from build123d import *

# Parameters (mm, degrees)
F0_W     = 20
F0_H     = 15
F0_W_2   = 75
F0_H_2   = 35
F0_W_3   = 15
F1_DEPTH = 60
F3_DEPTH = 50


with BuildPart() as f1:
    # F0 (on Top) → F1 (new body)
    with BuildSketch(Plane.XY):
        with Locations((45, 17.5)):
            Rectangle(F0_W, F0_H)
        with Locations((-2.5, 17.5)):
            Rectangle(F0_W_2, F0_H)
        with Locations((45, -7.5)):
            Rectangle(F0_W, F0_H_2)
        with Locations((-47.5, 17.5)):
            Rectangle(F0_W_3, F0_H)
        with Locations((-47.5, -7.5)):
            Rectangle(F0_W_3, F0_H_2)
    extrude(amount=F1_DEPTH)

    # F2 (on face) → F3 (cut)
    with BuildSketch(Plane.XZ.offset(25)):
        Polygon((55, 60), (-15, 60), (55, 20), align=None)
    extrude(amount=-F3_DEPTH, mode=Mode.SUBTRACT)


solid = f1.part
Source: CAD feature listing. Evaluate the final solid. Frame: model axes, mm. A direction names the side the tool comes from. Round coordinates to 2 decimals unless told otherwise and drop trailing zeros. Write each loop counter-clockwise with the first axis right and the second up, starting at its lowest first coordinate (ties: lowest second). Pieces come first, ordered by that corner, then holes. Notation, with made-up numbers: (9.5, -27.5) - (16.5, -27.5) arc R15 ccw to (16.5, -5.5) - close; hole circle Ø11 at (-6.75, -32.75). An arc over 180 degrees is marked (long way). Use CSV: the item, a comma, the result in double quotes. Start each with the question number.
(1) Set-up query: faces 1 (the face through (-1, 11, 0)), 2 (the face through (35, -8, 15)). Return all of +Z, -Z, +X, -X, +Y, -Y with unobstructed straight access to the full face (end or side cutting, diameter ignored); none if empty.
(2) Cut plane B-B, the plane z = 47. Return loops of the section in (x, y).
(3) Cut plane D-D, the plane z = 27. Return loops of the section in (x, y), and give its area (3 significant figures).
(4) Material intervals for probe 1 along X at (y, z) = (-9, 50); probe 2 along X at (y, z) = (-13.5, 24.5) (3 decimals); probe 3 along Y at (x, z) = (-20, 20), sorted ascending. Write a range as [from, to].
(5) First-contact query: pin 1 Ø10.5 at (y, z) = (-14, 30.5) entering from +X; pin 2 Ø1.5 at (x, z) = (-13.5, 42.5) entering from -Y. Flat tips, straight axial feed; report the tip coordinate or a pass-through.
(6) Cut plane A-A, the plane y = 6.5. Return loops of the section in (x, z), and give its area (3 significant figures).
(7) Mould query, pull axis X, two halves, no side actions, for faces 3 (the face through (-3, 10, 23)), 4 (the face through (-48, -25, 30)), 5 (the face through (-40, -8, 30)), 6 (the face through (55, 0, 10)). Classes: pulls with the +X half, pulls with the -X half, needs draft (parallel to the pull), parting line crosses it, or undercut.
(8) Cut plane C-C, the plane y = 13. Return loops of the section in (x, z).
Geometry says:
1,face 1,"-Z, +X, -X, +Y, -Y"
1,face 2,"+Z, -Z, -Y"
2,outline,"(-55, -25) - (-40, -25) - (-40, 10) - (7.75, 10) - (7.75, 25) - (-55, 25) - close"
3,outline,"(-55, -25) - (-40, -25) - (-40, 10) - (35, 10) - (35, -25) - (42.75, -25) - (42.75, 25) - (-55, 25) - close"
3,area,"2,260 mm²"
4,probe 1,"[-55, -40]"
4,probe 2,"[-55, -40], [35, 47.125]"
4,probe 3,"[10, 25]"
5,pin 1,"x = 45.81"
5,pin 2,"y = 10"
6,outline,"(-55, 0) - (-40, 0) - (-40, 60) - (-55, 60) - close; (35, 0) - (55, 0) - (55, 20) - (35, 31.43) - close"
6,area,"1,410 mm²"
7,face 3,"undercut"
7,face 4,"needs draft"
7,face 5,"undercut"
7,face 6,"pulls with the +X half"
8,outline,"(-55, 0) - (55, 0) - (55, 20) - (-15, 60) - (-55, 60) - close"
